```python
from build123d import *

# Parameters (mm, degrees)
SKETCH1_W           = 76.2
SKETCH1_H           = 101.6
BOSS_EXTRUDE1_DEPTH = 3.175
SKETCH2_R           = 14.2875
CUT_EXTRUDE1_DEPTH  = 28.575


with BuildPart() as part:
    # Sketch1 → Boss-Extrude1 (new body)
    with BuildSketch(Plane(origin=(0, 0, 0), x_dir=(1, 0, 0), z_dir=(0, 1, 0))):
        with Locations((38.1, -50.8)):
            Rectangle(SKETCH1_W, SKETCH1_H)
        Polygon((27.614248419, -19.05), (23.948074209, -12.7), (16.615725791, -12.7), (12.949551581, -19.05), (16.615725791, -25.4), (23.948074209, -25.4), align=None, mode=Mode.SUBTRACT)
        Polygon((55.9181, -11.717651581), (49.5681, -15.383825791), (49.5681, -22.716174209), (55.9181, -26.382348419), (62.2681, -22.716174209), (62.2681, -15.383825791), align=None, mode=Mode.SUBTRACT)
    extrude(amount=BOSS_EXTRUDE1_DEPTH)

    # Sketch2 → Cut-Extrude1 (cut)
    with BuildSketch(Plane(origin=(0, 3.175, 0), x_dir=(1, 0, 0), z_dir=(0, 1, 0))):
        with Locations(Location((20.2819, -19.05, 0), (0, 0, 270))):
            Circle(SKETCH2_R)
        with Locations(Location((55.9181, -19.05, 0), (0, 0, 270))):
            Circle(SKETCH2_R)
    extrude(amount=-CUT_EXTRUDE1_DEPTH, mode=Mode.SUBTRACT)


solid = part.part
```
Here's how the part is built. I have some questions about the finished solid (model axes, mm). Give positions to 0.01 mm unless a question says otherwise; leave off trailing zeros. Write each loop counter-clockwise with the first axis right and the second up, starting at its lowest first coordinate (ties: lowest second). Pieces come first, ordered by that corner, then holes. Notation, with made-up numbers: (39, -6) -> (71, -6) arc R8 cw to (71, 7) -> close; hole circle Ø9 at (-21, 32). An arc over 180 degrees is marked (long way). Write each question's results on one line, items separated by ' | '.
Item 1: Suppose I cut it at C-C on y = 1.5. Give the number of separate pieces and of enclosed holes in the cut face, plus the area to 3 significant figures.
Output:
separate pieces: 1 | enclosed holes: 2 | area: 6,460 mm^2
Item 2: If I drill on L1, parallel to X at y = 1.5, z = 19.05; L2, parallel to X at y = 1.9, z = 24; L3, parallel to Z at x = 18, y = 1.6, over which ranges is the centre line in solid material (lowest first)?
Output:
L1: x = 0 to 5.99, 34.57 to 41.63, 70.21 to 76.2 | L2: x = 0 to 6.88, 33.68 to 42.52, 69.32 to 76.2 | L3: z = 0 to 4.95, 33.15 to 101.6
Item 3: We'd pull the mould along X, two halves only. Please class faces 1 (the face through (14.81, 1.61, 32.25)), 2 (the face through (38, 2, 0)), 3 (the face through (0, 2, 52)): pulls with the +X half, pulls with the -X half, needs draft (parallel to the pull), parting line crosses it, or undercut.
Output:
face 1: undercut | face 2: needs draft | face 3: pulls with the -X half
Item 4: Suppose I cut it at B-B on x = 9.5. Write out the boundary of the cut face in (y, z) (3 decimals), plus the area to 3 significant figures.
Output:
outline: (0, 0) -> (3.175, 0) -> (3.175, 9.675) -> (0, 9.675) -> close; (0, 28.425) -> (3.175, 28.425) -> (3.175, 101.6) -> (0, 101.6) -> close | area: 263 mm^2
Item 5: Suppose I cut it at A-A on z = 19.05. Write out the boundary of the cut face in (x, y) (3 decimals), plus the area to 3 significant figures.
Output:
outline: (0, 0) -> (5.994, 0) -> (5.994, 3.175) -> (0, 3.175) -> close; (34.569, 0) -> (41.631, 0) -> (41.631, 3.175) -> (34.569, 3.175) -> close; (70.206, 0) -> (76.2, 0) -> (76.2, 3.175) -> (70.206, 3.175) -> close | area: 60.5 mm^2
Item 6: Suppose I cut it at D-D on x = 33. Write out the boundary of the cut face in (y, z) (3 decimals), plus the area to 3 significant figures.
Output:
outline: (0, 0) -> (3.175, 0) -> (3.175, 12.54) -> (0, 12.54) -> close; (0, 25.56) -> (3.175, 25.56) -> (3.175, 101.6) -> (0, 101.6) -> close | area: 281 mm^2
